Input: part model. Units: mm. Frame: model coordinates. A direction names the side the tool comes from. Give positions to 0.01 mm unless a question says otherwise; leave off trailing zeros. Write each loop counter-clockwise with the first axis right and the second up, starting at its lowest first coordinate (ties: lowest second). Pieces come first, ordered by that corner, then holes.
Autodesk Inventor part; units mm, degrees
ref_plane "YZ Plane" through (0, 0, 0) normal (1, 0, 0) x (0, 1, 0)
ref_plane "XZ Plane" through (0, 0, 0) normal (0, 1, 0) x (-1, 0, 0)
ref_plane "XY Plane" through (0, 0, 0) normal (0, 0, 1) x (1, 0, 0)
sketch "Sketch2" plane through (0, 0, 0) normal (0, 0, 1) x (1, 0, 0)
  line L0 (0, -3.6) -> (0, 21.6) construction
  line L1 (-7.2, 0) -> (1.2, 0) construction
  line L2 (0, 0) -> (-6, 0)
  line L3 (-6, 2) -> (-1.5, 2)
  line L4 (-1.5, 2) -> (-1.5, 4.114)
  line L5 (-1.5, 4.7135) -> (-1.5, 15)
  line L6 (-1.5, 15) -> (0, 15)
  line L7 (0, 0) -> (-6, 0)
  line L8 (-6, 2) -> (-6, 0)
  line L9 (-1.5, 3.3248) -> (-1.5, 5.5716)
  line L10 (0, 15) -> (0, 0)
  point P0 (-1.5, 4.114)
  dimension "d0" = 1.5
  dimension "d1" = 6
  dimension "d3" = 2
  dimension "HighRod" = 13
revolve "Revolution1" add sketch "Sketch2" angle 360 about axis through (0, -10, 0) along (0, 1, 0)
chamfer "Chamfer_top" [suppressed]
chamfer "Chamfer_bottom" distance 2 angle 45 1 edges at (6, 0, 0)
properties part number "P006" material "Aluminium"
Q1. Material intervals for line 1 along Y through (x, z) = (1, 2.25); line 2 along Y through (x, z) = (-4, -1.25); line 3 along X through (y, z) = (3, 0.5), sorted ascending.
Q2. Section C-C, the plane y = 12. Return the cut outline in (x, z).
Q3. Access query for faces 1 (the flat face through (0, 0, 0)), 2 (the cylindrical face through (1.5, 8.59, 0.07)). Directions: +Z, -Z, +X, -X, +Y, -Y. A direction counts if a zero-diameter tool reaches every point of the face in a straight line with its end or side. Return the directions, or none.
Q4. Pin query (flat end, axial travel): pin 1 (3 mm diameter, centred on x = -0.5, y = 10.5, fed in from -Z); pin 2 (5 mm diameter, centred on y = 11, z = 0, fed in from -X); pin 3 (2 mm diameter, centred on x = -2, y = 11, fed in from -Z). Return the tip coordinate at first contact, or that it passes through.
Solutions:
1. line 1: y = 0 to 2
1. line 2: y = 0.19 to 2
1. line 3: x = -1.41 to 1.41
2. outline: circle Ø3 at (0, 0)
3. face 1: +Z, -Z, +X, -X, -Y
3. face 2: +Y
4. pin 1: stops at z = -1.5
4. pin 2: stops at x = -1.5
4. pin 3: stops at z = -1.12
